Geometry check sheet. Reference: the model listing, model coordinates, mm. Coordinates: 2 decimals unless noted, no trailing zeros. Write each loop counter-clockwise with the first axis right and the second up, starting at its lowest first coordinate (ties: lowest second). Pieces come first, ordered by that corner, then holes. Notation, with made-up numbers: (6.5, 57) -> (35.5, 57) arc R13 cw to (35.5, 66) -> close; hole circle Ø11 at (-33.5, 72.5). An arc over 180 degrees is marked (long way). Answer as CSV lines item,"result".
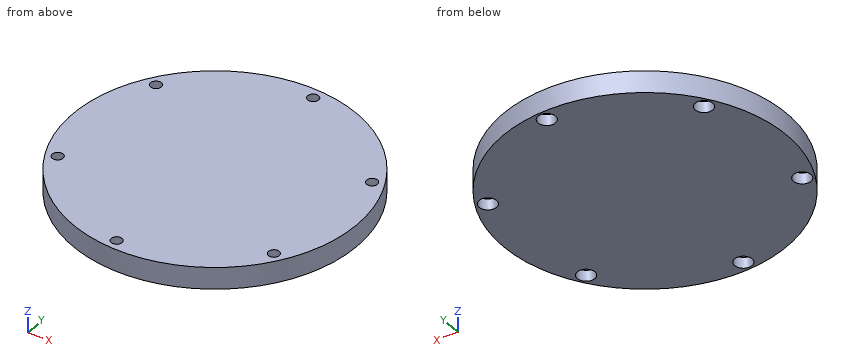
```python
from build123d import *

# Parameters (mm, degrees)
SKETCH_1_R          = 65
SKETCH_1_R_2        = 60
SKETCH_1_R_3        = 55
EXTRUDE_1_DEPTH     = 10
CUT_EXTRUDE_1_REACH = 94.466
SKETCH_2_R          = 2.5
SKETCH_3_R          = 4
SKETCH_3_R_2        = 2.5
CUT_EXTRUDE_2_DEPTH = 5


with BuildPart() as part:
    # 草图1 → 凸台-拉伸1 (new body)
    # profile 1 of 3: a face of its own
    with BuildSketch(Plane.XY):
        Circle(SKETCH_1_R)
        Circle(SKETCH_1_R_2, mode=Mode.SUBTRACT)
    # profile 2 of 3: a face of its own
    with BuildSketch(Plane.XY):
        Circle(SKETCH_1_R_2)
        Circle(SKETCH_1_R_3, mode=Mode.SUBTRACT)
    # profile 3 of 3: a face of its own
    with BuildSketch(Plane.XY):
        Circle(SKETCH_1_R_3)
    extrude(amount=EXTRUDE_1_DEPTH)

    # 草图2 → 切除-拉伸1 (cut, up to next)
    with BuildSketch(Plane(origin=(0, 0, 0), x_dir=(-1, 0, 0), z_dir=(0, 0, -1)), mode=Mode.PRIVATE) as cut_extrude_1_sk1:
        with Locations((-3.675520948, 59.887315399)):
            Circle(SKETCH_2_R)
    cut_extrude_1_tool1 = extrude(cut_extrude_1_sk1.sketch, amount=-CUT_EXTRUDE_1_REACH, mode=Mode.PRIVATE) & part.part
    # 草图2 → 切除-拉伸1 (cut, up to next)
    with BuildSketch(Plane(origin=(0, 0, 0), x_dir=(-1, 0, 0), z_dir=(0, 0, -1)), mode=Mode.PRIVATE) as cut_extrude_1_sk2:
        with Locations((50.026176026, 33.126752213)):
            Circle(SKETCH_2_R)
    cut_extrude_1_tool2 = extrude(cut_extrude_1_sk2.sketch, amount=-CUT_EXTRUDE_1_REACH, mode=Mode.PRIVATE) & part.part
    # 草图2 → 切除-拉伸1 (cut, up to next)
    with BuildSketch(Plane(origin=(0, 0, 0), x_dir=(-1, 0, 0), z_dir=(0, 0, -1)), mode=Mode.PRIVATE) as cut_extrude_1_sk3:
        with Locations((53.701696975, -26.760563186)):
            Circle(SKETCH_2_R)
    cut_extrude_1_tool3 = extrude(cut_extrude_1_sk3.sketch, amount=-CUT_EXTRUDE_1_REACH, mode=Mode.PRIVATE) & part.part
    # 草图2 → 切除-拉伸1 (cut, up to next)
    with BuildSketch(Plane(origin=(0, 0, 0), x_dir=(-1, 0, 0), z_dir=(0, 0, -1)), mode=Mode.PRIVATE) as cut_extrude_1_sk4:
        with Locations((3.675520948, -59.887315399)):
            Circle(SKETCH_2_R)
    cut_extrude_1_tool4 = extrude(cut_extrude_1_sk4.sketch, amount=-CUT_EXTRUDE_1_REACH, mode=Mode.PRIVATE) & part.part
    # 草图2 → 切除-拉伸1 (cut, up to next)
    with BuildSketch(Plane(origin=(0, 0, 0), x_dir=(-1, 0, 0), z_dir=(0, 0, -1)), mode=Mode.PRIVATE) as cut_extrude_1_sk5:
        with Locations((-50.026176026, -33.126752213)):
            Circle(SKETCH_2_R)
    cut_extrude_1_tool5 = extrude(cut_extrude_1_sk5.sketch, amount=-CUT_EXTRUDE_1_REACH, mode=Mode.PRIVATE) & part.part
    # 草图2 → 切除-拉伸1 (cut, up to next)
    with BuildSketch(Plane(origin=(0, 0, 0), x_dir=(-1, 0, 0), z_dir=(0, 0, -1)), mode=Mode.PRIVATE) as cut_extrude_1_sk6:
        with Locations((-53.701696975, 26.760563186)):
            Circle(SKETCH_2_R)
    cut_extrude_1_tool6 = extrude(cut_extrude_1_sk6.sketch, amount=-CUT_EXTRUDE_1_REACH, mode=Mode.PRIVATE) & part.part
    add(cut_extrude_1_tool1.solids().sort_by_distance((3.675521, 59.887315, 0))[0], mode=Mode.SUBTRACT)
    add(cut_extrude_1_tool2.solids().sort_by_distance((-50.026176, 33.126752, 0))[0], mode=Mode.SUBTRACT)
    add(cut_extrude_1_tool3.solids().sort_by_distance((-53.701697, -26.760563, 0))[0], mode=Mode.SUBTRACT)
    add(cut_extrude_1_tool4.solids().sort_by_distance((-3.675521, -59.887315, 0))[0], mode=Mode.SUBTRACT)
    add(cut_extrude_1_tool5.solids().sort_by_distance((50.026176, -33.126752, 0))[0], mode=Mode.SUBTRACT)
    add(cut_extrude_1_tool6.solids().sort_by_distance((53.701697, 26.760563, 0))[0], mode=Mode.SUBTRACT)

    # 草图3 → 切除-拉伸2 (cut)
    # profile 1 of 6: a face of its own
    with BuildSketch(Plane(origin=(0, 0, 0), x_dir=(-1, 0, 0), z_dir=(0, 0, -1))):
        with Locations((-3.675520948, 59.887315399)):
            Circle(SKETCH_3_R)
        with Locations((-3.675520948, 59.887315399)):
            Circle(SKETCH_3_R_2, mode=Mode.SUBTRACT)
    # profile 2 of 6: a face of its own
    with BuildSketch(Plane(origin=(0, 0, 0), x_dir=(-1, 0, 0), z_dir=(0, 0, -1))):
        with Locations((50.026176026, 33.126752213)):
            Circle(SKETCH_3_R)
    # profile 3 of 6: a face of its own
    with BuildSketch(Plane(origin=(0, 0, 0), x_dir=(-1, 0, 0), z_dir=(0, 0, -1))):
        with Locations((53.701696975, -26.760563186)):
            Circle(SKETCH_3_R)
    # profile 4 of 6: a face of its own
    with BuildSketch(Plane(origin=(0, 0, 0), x_dir=(-1, 0, 0), z_dir=(0, 0, -1))):
        with Locations((3.675520948, -59.887315399)):
            Circle(SKETCH_3_R)
    # profile 5 of 6: a face of its own
    with BuildSketch(Plane(origin=(0, 0, 0), x_dir=(-1, 0, 0), z_dir=(0, 0, -1))):
        with Locations((-50.026176026, -33.126752213)):
            Circle(SKETCH_3_R)
    # profile 6 of 6: a face of its own
    with BuildSketch(Plane(origin=(0, 0, 0), x_dir=(-1, 0, 0), z_dir=(0, 0, -1))):
        with Locations((-53.701696975, 26.760563186)):
            Circle(SKETCH_3_R)
    extrude(amount=-CUT_EXTRUDE_2_DEPTH, mode=Mode.SUBTRACT)


solid = part.part
```
Item 1: Cross-section at A-A, the plane z = 3.25. Record the cut outline in (x, y), plus the area to 3 significant figures.
Responses:
outline,"circle Ø130 at (0, 0); hole circle Ø8 at (-53.7, -26.76); hole circle Ø8 at (-50.03, 33.13); hole circle Ø8 at (-3.68, -59.89); hole circle Ø8 at (3.68, 59.89); hole circle Ø8 at (50.03, -33.13); hole circle Ø8 at (53.7, 26.76)"
area,"13,000 mm2"
Item 2: Thickness scan on probe 1 along Y at (x, z) = (6.5, 3.5); probe 2 along Y at (x, z) = (2, 5.25); probe 3 along X at (y, z) = (-25, 4). Record the ranges inside material, lowest first.
Responses:
probe 1,"y = -64.67 to 57.05, 62.72 to 64.67"
probe 2,"y = -64.97 to 58.03, 61.74 to 64.97"
probe 3,"x = -60 to -57.29, -50.11 to 60"
Item 3: Cross-section at B-B, the plane y = 12. Record the cut outline in (x, z).
Responses:
outline,"(-63.88, 0) -> (63.88, 0) -> (63.88, 10) -> (-63.88, 10) -> close"
Item 4: Depth check by flat-ended pin: pin 1 Ø9 at (x, y) = (2.5, 60.5) entering from -Z; pin 2 Ø5 at (x, z) = (-40.5, 1) entering from +Y; pin 3 Ø1 at (y, z) = (-25, 7.5) entering from -X; pin 4 Ø4 at (x, z) = (-41, 8.5) entering from +Y. Enter the tip coordinate at first touch or a pass-through.
Responses:
pin 1,"stops at z = 0"
pin 2,"stops at y = 52.74"
pin 3,"stops at x = -60.21"
pin 4,"stops at y = 52"
